Study the drawing (mm; zero at the part's minimum x, y, z) and answer. A direction names the side the tool comes from. Coordinates: 2 decimals unless noted, no trailing zeros. Write each loop counter-clockwise with the first axis right and the second up, starting at its lowest first coordinate (ties: lowest second). Pieces come first, ordered by that corner, then holes. Notation, with made-up numbers: (-38, -26) - (-32, -26) arc R4 ccw to (-32, -20) - close; hole circle Ø7 at (9, -13). An arc over 180 degrees is marked (long way). One line per item, written item: value.
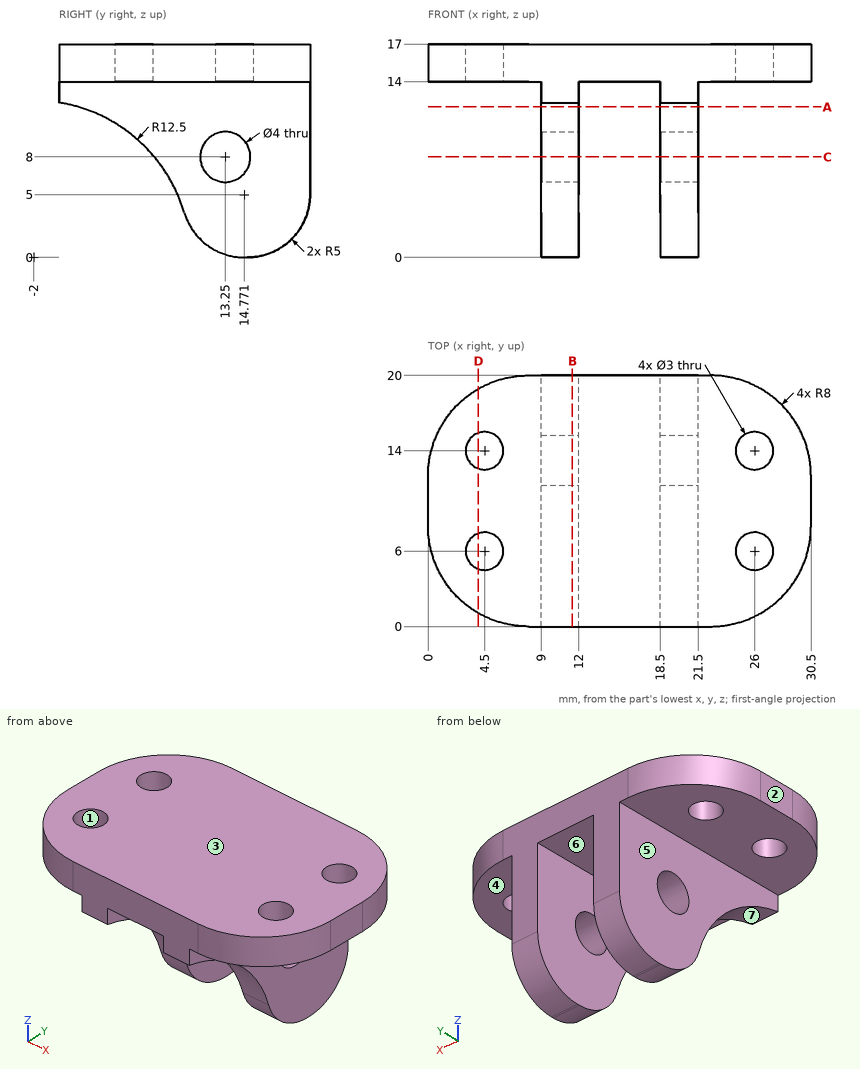
Item 1: Section D-D, the plane x = 4 is taken. Determine the outline of the cut face in (y, z) (1 decimal), then the cut area to 3 significant figures.
Evaluation:
outline: (1.1, 14) - (4.6, 14) - (4.6, 17) - (1.1, 17) - close; (7.4, 14) - (12.6, 14) - (12.6, 17) - (7.4, 17) - close; (15.4, 14) - (18.9, 14) - (18.9, 17) - (15.4, 17) - close
area: 36.6 mm2
Item 2: Section B-B, the plane x = 11.5 is taken. Determine the outline of the cut face in (y, z).
Evaluation:
outline: (0, 12.34) arc R12.5 cw to (9.98, 3.57) arc R5 ccw to (14.77, 0) - (15, 0) arc R5 ccw to (20, 5) - (20, 17) - (0, 17) - close; hole circle Ø4 at (13.25, 8)
Item 3: Determine the mould class of the marked faces 1, 2 and 3 for opening direction X: +X half, -X half, draft (parallel to the pull), parting line (faces both ways), or undercut.
Evaluation:
face 1: undercut
face 2: -X half
face 3: draft
Item 4: Section A-A, the plane z = 12 is taken. Determine the outline of the cut face in (x, y), then the cut area to 3 significant figures.
Evaluation:
outline: (9, 1.5) - (12, 1.5) - (12, 20) - (9, 20) - close; (18.5, 1.5) - (21.5, 1.5) - (21.5, 20) - (18.5, 20) - close
area: 111 mm2
Item 5: Which of the six approach directions +Z, -Z, +X, -X, +Y, -Y give full straight-line access (tool end or side, diameter ignored) to the marked faces 4, 5, 6 and 7?
Evaluation:
face 4: -Z, +X, +Y, -Y
face 5: -Z, -X, +Y, -Y
face 6: -Z, +Y, -Y
face 7: -Z, +X, -X, -Y
Item 6: Section C-C, the plane z = 8 is taken. Give the number of separate pieces and of enclosed holes in the cut face.
Evaluation:
separate pieces: 4
enclosed holes: 0
Item 7: Given pin 1 (10 mm diameter, centred on x = 5, y = 8.5, fed in from -Z); pin 2 (1 mm diameter, centred on y = 6.5, z = 15, fed in from -X); pin 3 (1 mm diameter, centred on y = 10, z = 4, fed in from -X); pin 4 (2.5 mm diameter, centred on x = 4.5, y = 14, fed in from -Z), each flat-ended and moving along its own axis, determine where each tip first touches the part or whether it passes through.
Evaluation:
pin 1: stops at z = 1.22
pin 2: stops at x = 0.06
pin 3: stops at x = 9
pin 4: passes through
Item 8: Consider probe 1 along X at (y, z) = (17, 9.25); probe 2 along Y at (x, z) = (26, 15.6) (1 decimal); probe 3 along Z at (x, y) = (5, 3.5). Determine where each line is inside the solid, lowest interval first.
Evaluation:
probe 1: x = 9 to 12, 18.5 to 21.5
probe 2: y = 0.8 to 4.5, 7.5 to 12.5, 15.5 to 19.2
probe 3: z = 14 to 17
